Input: part model. Units: mm. Frame: model coordinates. Face numbers are marked on the shaded views. A direction names the side the tool comes from. Coordinates: 2 decimals unless noted, no trailing zeros. Write each loop counter-clockwise with the first axis right and the second up, starting at its lowest first coordinate (ties: lowest second). Pieces come first, ordered by that corner, then holes. Notation, with made-up numbers: M 80,53.25 L 84,53.25 A22 ccw 84,64.25 Z; hole C 63,9.25 d5. An arc over 180 degrees is marked long. Use one line per item in the form item = value.
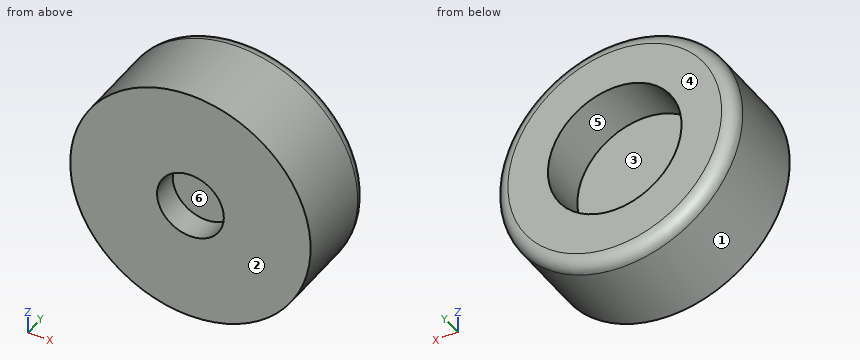
from build123d import *

# Parameters (mm, degrees)
SKETCH1_R           = 11.43
BOSS_EXTRUDE1_DEPTH = 8.89
SKETCH2_R           = 6.35
CUT_EXTRUDE1_DEPTH  = 4.7625
FILLET4_R           = 1.27
SKETCH3_R           = 3.175
CUT_EXTRUDE2_DEPTH  = 2.54


with BuildPart() as part:
    # Sketch1 → Boss-Extrude1 (new body)
    with BuildSketch(Plane(origin=(0, 0, 0), x_dir=(1, 0, 0), z_dir=(0, 1, 0))):
        with Locations(Location((0, 0, 0), (0, 0, 270))):
            Circle(SKETCH1_R)
    extrude(amount=BOSS_EXTRUDE1_DEPTH)

    # Sketch2 → Cut-Extrude1 (cut)
    with BuildSketch(Plane(origin=(0, 8.89, 0), x_dir=(1, 0, 0), z_dir=(0, 1, 0))):
        with Locations(Location((0, 0, 0), (0, 0, 270))):
            Circle(SKETCH2_R)
    extrude(amount=-CUT_EXTRUDE1_DEPTH, mode=Mode.SUBTRACT)

    # Fillet4
    fillet4_edges = [part.edges().sort_by_distance(p)[0] for p in [
        (0, 8.89, -11.43),
    ]]
    fillet(fillet4_edges, radius=FILLET4_R)

    # Sketch3 → Cut-Extrude2 (cut)
    with BuildSketch(Plane.XZ):
        with Locations(Location((0, 0, 0), (0, 0, 270))):
            Circle(SKETCH3_R)
    extrude(amount=-CUT_EXTRUDE2_DEPTH, mode=Mode.SUBTRACT)


solid = part.part
(1) Pull-direction query (Z, two-part tool) for the marked faces 1, 2 and 3; classes: pulls with the +Z half, pulls with the -Z half, needs draft (parallel to the pull), parting line crosses it, or undercut.
Computed:
face_1 = parting line crosses it
face_2 = needs draft
face_3 = undercut
(2) Section query C-C on y = 3.25. Return the cut outline in (x, z), plus the area to 3 significant figures.
Computed:
outline = C 0,0 d22.86
area = 410 mm^2
(3) First-contact query: pin 1 Ø4 at (x, z) = (3, -2) entering from +Y; pin 2 Ø7 at (x, z) = (-1.5, 1.5) entering from -Y; pin 3 Ø1 at (y, z) = (3, 2.5) entering from +X; pin 4 Ø4 at (x, z) = (0, 0) entering from -Y. Flat tips, straight axial feed; report the tip coordinate or a pass-through.
Computed:
pin_1 = 4.13
pin_2 = 0
pin_3 = 11.25
pin_4 = 2.54
(4) Line query: probe 1 along X at (y, z) = (1.3, 0) (3 decimals); probe 2 along Y at (x, z) = (2.5, -0.75); probe 3 along X at (y, z) = (6.25, 0). Output: solid intervals per line, ascending.
Computed:
probe_1 = -11.43 to -3.175, 3.175 to 11.43
probe_2 = 2.54 to 4.13
probe_3 = -11.43 to -6.35, 6.35 to 11.43
(5) Section query D-D on y = 8. Return the cut outline in (x, z), plus the area to 3 significant figures.
Computed:
outline = C 0,0 d22.74; hole C 0,0 d12.7
area = 280 mm^2
(6) Set-up query: the marked faces 4, 5 and 6. Return all of +Z, -Z, +X, -X, +Y, -Y with unobstructed straight access to the full face (end or side cutting, diameter ignored); none if empty.
Computed:
face_4 = +Z, -Z, +X, -X, +Y
face_5 = +Y
face_6 = -Y
